CAD build for the part. Positions are in the model's coordinates, mm. Round coordinates to 2 decimals unless told otherwise and drop trailing zeros. Write each loop counter-clockwise with the first axis right and the second up, starting at its lowest first coordinate (ties: lowest second). Pieces come first, ordered by that corner, then holes. Notation, with made-up numbers: (-21, 69) - (3, 69) arc R19 cw to (3, 75) - close; hole circle Ø3 at (66, -15.75). An arc over 180 degrees is marked (long way). Put each result on its own line as item: value. Start each with the question number.
Item 1: Cut at A-A (z = 2). Give the cut face in (x, y) (3 decimals), and give its area (3 significant figures).
Item 2: Cut at B-B (x = -53.5). Give the cut face in (y, z), and give its area (3 significant figures).
Item 3: Drill centre lines: line 1 (X direction, y = -10.5, z = 3) (3 decimals); line 2 (X direction, y = 8, z = 2.75) (3 decimals); line 3 (Y direction, x = 52, z = 1.5). Where is each one in solid material? Low to high. Write a range as from..to.
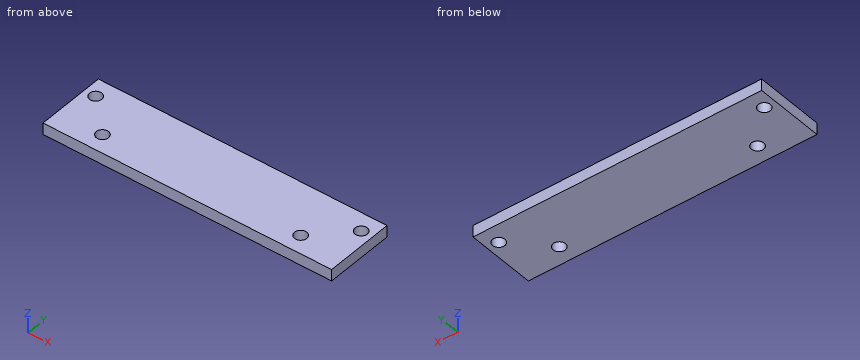
```python
from build123d import *

# Parameters (mm, degrees)
SKETCH1_W               = 158.75
SKETCH1_H               = 38.1
BOSS_EXTRUDE1_DEPTH     = 6.35
F_1_4_CLEARANCE_HOLE1_D = 6.7564


with BuildPart() as part:
    # Sketch1 → Boss-Extrude1 (new body)
    with BuildSketch(Plane.XY):
        Rectangle(SKETCH1_W, SKETCH1_H)
    extrude(amount=BOSS_EXTRUDE1_DEPTH)

    # 1/4 Clearance Hole1 (through all)
    with Locations(Plane.XY.offset(6.35)):
        with Locations((-73.025, 9.249663805), (-54.525672391, -9.249663805)):
            f_1_4_clearance_hole1 = Hole(F_1_4_CLEARANCE_HOLE1_D / 2)

    # Mirror1: 1/4 Clearance Hole1 across plane
    add(f_1_4_clearance_hole1.mirror(Plane(origin=(0, 0, 0), x_dir=(0, 0, 1), z_dir=(1, 0, 0))), mode=Mode.SUBTRACT)


solid = part.part
```
Output values:
1. outline: (-79.375, -19.05) - (79.375, -19.05) - (79.375, 19.05) - (-79.375, 19.05) - close; hole circle Ø6.756 at (-73.025, 9.25); hole circle Ø6.756 at (-54.526, -9.25); hole circle Ø6.756 at (54.526, -9.25); hole circle Ø6.756 at (73.025, 9.25)
1. area: 5,900 mm2
2. outline: (-19.05, 0) - (-12.47, 0) - (-12.47, 6.35) - (-19.05, 6.35) - close; (-6.03, 0) - (19.05, 0) - (19.05, 6.35) - (-6.03, 6.35) - close
2. area: 201 mm2
3. line 1: -79.375..-57.664, -51.387..51.387, 57.664..79.375
3. line 2: -79.375..-76.164, -69.886..69.886, 76.164..79.375
3. line 3: -19.05..-11.49, -7.01..19.05
